from build123d import *

# Parameters (mm, degrees)
SKETCH_1_R      = 2.5
EXTRUDE_1_DEPTH = 4


with BuildPart() as part:
    # 草图1 → 凸台-拉伸1 (new body)
    with BuildSketch(Plane(origin=(0, 0, 0), x_dir=(1, 0, 0), z_dir=(0, 1, 0))):
        with BuildLine():
            Line((-20.346989949, 35.242020373), (-15.461646096, 26.780356607))
            ThreePointArc((-15.461646096, 26.780356607), (-12.365785271, 24.159967367), (-8.310161545, 24.10790773))
            ThreePointArc((-8.310161545, 24.10790773), (22.083647797, -12.75), (-25.033141298, -4.857142857))
            ThreePointArc((-25.033141298, -4.857142857), (-27.10603813, -1.370899501), (-30.923292192, 0))
            Line((-30.923292192, 0), (-40.693979899, 0))
            ThreePointArc((-40.693979899, 0), (-44.438895151, 1.687054218), (-45.656660374, 5.609756098))
            ThreePointArc((-45.656660374, 5.609756098), (-39.837168574, 23), (-27.686521477, 36.734949687))
            ThreePointArc((-27.686521477, 36.734949687), (-23.680479385, 37.641685008), (-20.346989949, 35.242020373))
        make_face()
        with Locations(Location((0, 11, 0), (0, 0, 270))):
            Circle(SKETCH_1_R, mode=Mode.SUBTRACT)
        with Locations(Location((9.462063016, 5.609756098, 0), (0, 0, 270))):
            Circle(SKETCH_1_R, mode=Mode.SUBTRACT)
        with Locations(Location((9.526279442, -5.5, 0), (0, 0, 270))):
            Circle(SKETCH_1_R, mode=Mode.SUBTRACT)
        with Locations(Location((0, -11, 0), (0, 0, 270))):
            Circle(SKETCH_1_R, mode=Mode.SUBTRACT)
        with Locations(Location((-9.526279442, -5.5, 0), (0, 0, 270))):
            Circle(SKETCH_1_R, mode=Mode.SUBTRACT)
        with Locations(Location((-9.526279442, 5.5, 0), (0, 0, 270))):
            Circle(SKETCH_1_R, mode=Mode.SUBTRACT)
    extrude(amount=EXTRUDE_1_DEPTH)


solid = part.part
Model file for the job. Use its own axes, mm. A direction names the side the tool comes from. Give positions to 0.01 mm unless a question says otherwise; leave off trailing zeros. Loops run counter-clockwise (first coordinate to the right, second up) from the corner with the lowest first, then second, coordinate; pieces in that order, holes last.
1) Saw through at A-A (x = 0). Write the cut outline in (y, z).
2) Tool access for faces 5 (the flat face through (-36, 2, 0)), 6 (the flat face through (-17.94, 1.97, -31.07)): list every direction of +Z, -Z, +X, -X, +Y, -Y with a clear straight run to the whole face (end or side of a thin tool).
3) Wall check: line 1 (Z direction, x = 9, y = 3.75); line 2 (Z direction, x = -10.5, y = 1.5); line 3 (X direction, y = 2.85, z = -6.5) (3 decimals). Give the ranges that are in metal, low to high.
4) Saw through at B-B (z = -9.5). Write the cut outline in (x, y).
5) Saw through at C-C (y = 0.8). Write the cut outline in (x, z), plus the area to 3 significant figures.
6) Pull direction X, two halves, no side cores. Call faces 1 (the cylindrical face through (10.277, 1.972, 7.885)), 2 (the cylindrical face through (0.1, 2, -13.5)), 3 (the cylindrical face through (-39.966, 1.972, -22.776)), 4 (the cylindrical face through (-23.739, 1.972, -37.653)): +X half, -X half, draft (parallel to the pull), parting line (faces both ways), or undercut.
7) Saw through at D-D (x = 8). Write the cut outline in (y, z), plus the area to 3 significant figures.
8) Flat gauge pins, fed straight in: pin 1 Ø6 at (x, z) = (-9.53, 5.5) entering from +Y; pin 2 Ø3 at (x, z) = (0, 11) entering from -Y; pin 3 Ø1.2 at (x, y) = (-37, 1.5) entering from +Z. Where does each tip first touch, or does it go through?
Answer block:
1. outline: (0, -25.5) - (4, -25.5) - (4, -13.5) - (0, -13.5) - close; (0, -8.5) - (4, -8.5) - (4, 8.5) - (0, 8.5) - close; (0, 13.5) - (4, 13.5) - (4, 25.5) - (0, 25.5) - close
2. face 5: +Z, -X, +Y, -Y
2. face 6: -Z, +X, +Y, -Y
3. line 1: z = -23.86 to -8.07, -3.15 to 3.06, 7.94 to 23.86
3. line 2: z = -23.78 to -7.8, -3.2 to 3.2, 7.8 to 23.24
3. line 3: x = -45.538 to -11.818, -7.235 to 7.126, 11.798 to 24.658
4. outline: (-45.01, 0) - (-2, 0) - (-2, 4) - (-45.01, 4) - close; (2, 0) - (23.66, 0) - (23.66, 4) - (2, 4) - close
5. outline: (-45.66, -5.61) arc R46 ccw to (-27.69, -36.73) arc R5 ccw to (-20.35, -35.24) - (-15.46, -26.78) arc R6 cw to (-8.31, -24.11) arc R25.5 ccw (long way) to (-25.03, 4.86) arc R6 cw to (-30.92, 0) - (-40.69, 0) arc R5 ccw to start; hole circle Ø5 at (-9.53, -5.5); hole circle Ø5 at (-9.53, 5.5); hole circle Ø5 at (0, -11); hole circle Ø5 at (0, 11); hole circle Ø5 at (9.46, -5.61); hole circle Ø5 at (9.53, 5.5)
5. area: 2,690 mm2
6. face 1: undercut
6. face 2: undercut
6. face 3: -X half
6. face 4: parting line
7. outline: (0, -24.21) - (4, -24.21) - (4, -7.64) - (0, -7.64) - close; (0, -3.58) - (4, -3.58) - (4, 3.52) - (0, 3.52) - close; (0, 7.48) - (4, 7.48) - (4, 24.21) - (0, 24.21) - close
7. area: 162 mm2
8. pin 1: stops at y = 4
8. pin 2: passes through
8. pin 3: stops at z = 0
